from build123d import *

# Parameters (mm, degrees)
F1_DEPTH     = 6
F3_DEPTH     = 4.8
F4_T1_DEPTH  = 13.92
F4_T3_DEPTH  = 5.5
F4_T6_ANGLE  = 90
F4_T8_ANGLE  = 90
F4_T10_ANGLE = 90
F4_T12_ANGLE = 90
F4_T14_ANGLE = 90
F4_T16_ANGLE = 90
F4_T18_ANGLE = 90
F4_T20_ANGLE = 90
F5_W         = 5.9125532862
F5_H         = 4.6649316102
F6_DEPTH     = 1
F7_W         = 5.9137202334
F7_H         = 4.6533403695
F8_DEPTH     = 1


# Not quite as in the source:
# - a fillet or chamfer that OpenCascade refuses, or shapes differently, is made with other operations: its cross-section is extruded or revolved along the edge and cut away or added


with BuildPart() as f1:
    # F0 (on Top) → F1 (new body)
    with BuildSketch(Plane.XY):
        with BuildLine():
            Line((6.96, 5.75), (-6.96, 5.75))
            ThreePointArc((-6.96, 5.75), (-9.0813203436, 4.8713203436), (-9.96, 2.75))
            Line((-9.96, 2.75), (-9.96, -2.75))
            ThreePointArc((-9.96, -2.75), (-9.0813203436, -4.8713203436), (-6.96, -5.75))
            Line((-6.96, -5.75), (6.96, -5.75))
            ThreePointArc((6.96, -5.75), (9.0813203436, -4.8713203436), (9.96, -2.75))
            Line((9.96, -2.75), (9.96, 2.75))
            ThreePointArc((9.96, 2.75), (9.0813203436, 4.8713203436), (6.96, 5.75))
        make_face()
    extrude(amount=F1_DEPTH)

    # F2 (on face) → F3 (cut)
    with BuildSketch(Plane.XY.offset(6)):
        Polygon((2.95, 5.1095498823), (-2.95, 5.1095498823), (-5.9, 0), (-2.95, -5.1095498823), (2.95, -5.1095498823), (5.9, 0), align=None)
    extrude(amount=-F3_DEPTH, mode=Mode.SUBTRACT)

    # F4: chamfer of 1 on 2 edges, made by hand

    # F4_s2 → F4_t1 (cut)
    with BuildSketch(Plane.YZ.offset(-6.96)):
        Polygon((5.75, 5), (4.75, 6), (5.75, 6), align=None)
        Polygon((5.75, 1), (4.75, 0), (5.75, 0), align=None)
        Polygon((-4.75, 0), (-5.75, 1), (-5.75, 0), align=None)
        Polygon((-4.75, 6), (-5.75, 5), (-5.75, 6), align=None)
    extrude(amount=F4_T1_DEPTH, mode=Mode.SUBTRACT)

    # F4_s4 → F4_t3 (cut)
    with BuildSketch(Plane.XZ.offset(-2.75)):
        Polygon((-8.96, 0), (-9.96, 1), (-9.96, 0), align=None)
        Polygon((8.96, 0), (9.96, 1), (9.96, 0), align=None)
        Polygon((-8.96, 6), (-9.96, 5), (-9.96, 6), align=None)
        Polygon((8.96, 6), (9.96, 5), (9.96, 6), align=None)
    extrude(amount=F4_T3_DEPTH, mode=Mode.SUBTRACT)

    # F4_s5 → F4_t6 (revolve, cut)
    with BuildSketch(Plane.XZ.offset(-2.75)):
        Polygon((9.96, 1), (8.96, 0), (9.96, 0), align=None)
    revolve(axis=Axis((6.96, 2.75, 0), (0, 0, 1)), revolution_arc=F4_T6_ANGLE, mode=Mode.SUBTRACT)

    # F4_s7 → F4_t8 (revolve, cut)
    with BuildSketch(Plane.YZ.offset(-6.96)):
        Polygon((5.75, 1), (4.75, 0), (5.75, 0), align=None)
    revolve(axis=Axis((-6.96, 2.75, 0), (0, 0, 1)), revolution_arc=F4_T8_ANGLE, mode=Mode.SUBTRACT)

    # F4_s9 → F4_t10 (revolve, cut)
    with BuildSketch(Plane.XZ.offset(2.75)):
        Polygon((-8.96, 0), (-9.96, 1), (-9.96, 0), align=None)
    revolve(axis=Axis((-6.96, -2.75, 0), (0, 0, 1)), revolution_arc=F4_T10_ANGLE, mode=Mode.SUBTRACT)

    # F4_s11 → F4_t12 (revolve, cut)
    with BuildSketch(Plane.YZ.offset(6.96)):
        Polygon((-4.75, 0), (-5.75, 1), (-5.75, 0), align=None)
    revolve(axis=Axis((6.96, -2.75, 0), (0, 0, 1)), revolution_arc=F4_T12_ANGLE, mode=Mode.SUBTRACT)

    # F4_s13 → F4_t14 (revolve, cut)
    with BuildSketch(Plane.XZ.offset(-2.75)):
        Polygon((9.96, 5), (8.96, 6), (9.96, 6), align=None)
    revolve(axis=Axis((6.96, 2.75, 6), (0, 0, 1)), revolution_arc=F4_T14_ANGLE, mode=Mode.SUBTRACT)

    # F4_s15 → F4_t16 (revolve, cut)
    with BuildSketch(Plane.YZ.offset(-6.96)):
        Polygon((5.75, 5), (4.75, 6), (5.75, 6), align=None)
    revolve(axis=Axis((-6.96, 2.75, 6), (0, 0, 1)), revolution_arc=F4_T16_ANGLE, mode=Mode.SUBTRACT)

    # F4_s17 → F4_t18 (revolve, cut)
    with BuildSketch(Plane.XZ.offset(2.75)):
        Polygon((-8.96, 6), (-9.96, 5), (-9.96, 6), align=None)
    revolve(axis=Axis((-6.96, -2.75, 6), (0, 0, 1)), revolution_arc=F4_T18_ANGLE, mode=Mode.SUBTRACT)

    # F4_s19 → F4_t20 (revolve, cut)
    with BuildSketch(Plane.YZ.offset(6.96)):
        Polygon((-4.75, 6), (-5.75, 5), (-5.75, 6), align=None)
    revolve(axis=Axis((6.96, -2.75, 6), (0, 0, 1)), revolution_arc=F4_T20_ANGLE, mode=Mode.SUBTRACT)

    # F5 (on face) → F6 (cut)
    with BuildSketch(Plane.XZ.offset(5.75)):
        with Locations((0.007480965, 3.3324658051)):
            Rectangle(F5_W, F5_H)
    extrude(amount=-F6_DEPTH, mode=Mode.SUBTRACT)

    # F7 (on face) → F8 (cut)
    with BuildSketch(Plane(origin=(0, 5.75, 0), x_dir=(-1, 0, 0), z_dir=(0, 1, 0))):
        with Locations((0.0472323736, 3.3266701847)):
            Rectangle(F7_W, F7_H)
    extrude(amount=-F8_DEPTH, mode=Mode.SUBTRACT)


solid = f1.part
Work out the finished part from the listing and answer in its coordinate system (mm). A direction names the side the tool comes from. Round coordinates to 2 decimals unless told otherwise and drop trailing zeros. Loops run counter-clockwise (first coordinate to the right, second up) from the corner with the lowest first, then second, coordinate; pieces in that order, holes last. Notation, with made-up numbers: (49, -3.5) - (56, -3.5) arc R10 ccw to (56, 2.5) - close; hole circle Ø11 at (-12.5, 33.5). An arc over 180 degrees is marked (long way). One line per item, written item: value.
Q1. The mould has two halves that part along X. Classify faces 4 (the flat face through (0, 5, 1)), 5 (the flat face through (-2.949, -5.4, 3.3)), 6 (the conical face through (8.6, -4.5, 5.6)), 7 (the cylindrical face through (-9.06, 4.89, 2.97)): +X half, -X half, draft (parallel to the pull), parting line (faces both ways), or undercut.
Check values:
face 4: undercut
face 5: undercut
face 6: +X half
face 7: -X half
Q2. Find section B-B on x = -1. Give the vertices of the cut face in (y, z).
Check values:
outline: (-5.75, 1) - (-4.75, 0) - (4.75, 0) - (5.75, 1) - (4.75, 1) - (4.75, 1.2) - (-4.75, 1.2) - (-4.75, 1) - close
Q3. Straight lines are drawn through the part: probe 1 along X at (y, z) = (-2, 2.65); probe 2 along X at (y, z) = (-1.5, 2.6); probe 3 along Z at (x, y) = (3, -4). For each, find the intervals that lie inside material, in ascending order.
Check values:
probe 1: -9.96 to -4.75, 4.75 to 9.96
probe 2: -9.96 to -5.03, 5.03 to 9.96
probe 3: 0 to 1.2
Q4. Find section D-D on y = 1.5. Give the vertices of the cut face in (x, z), and give its area (3 significant figures).
Check values:
outline: (-9.96, 1) - (-8.96, 0) - (8.96, 0) - (9.96, 1) - (9.96, 5) - (8.96, 6) - (5.03, 6) - (5.03, 1.2) - (-5.03, 1.2) - (-5.03, 6) - (-8.96, 6) - (-9.96, 5) - close
area: 69.2 mm2
Q5. For faces 1 (the flat face through (4.4, -2.6, 3.6)), 2 (the flat face through (2.964, -5.4, 3.3)), 3 (the flat face through (-5, -5.75, 3)), determine the directions among +Z, -Z, +X, -X, +Y, -Y from which every point of the face is accessible in a straight line to the end or side of a thin tool.
Check values:
face 1: +Z
face 2: +Z, -Y
face 3: +Z, -Z, +X, -X, -Y
Q6. Each of these flat-tipped pins is pushed along its axis until it touches: pin 1 Ø0.8 at (y, z) = (-5, 4) entering from +X; pin 2 Ø0.5 at (y, z) = (5.5, 3) entering from -X; pin 3 Ø1.1 at (x, y) = (0.5, 5.5) entering from +Z. Where does it stop, or does it pass through?
Check values:
pin 1: x = 9.32
pin 2: x = -8.62
pin 3: z = 1
